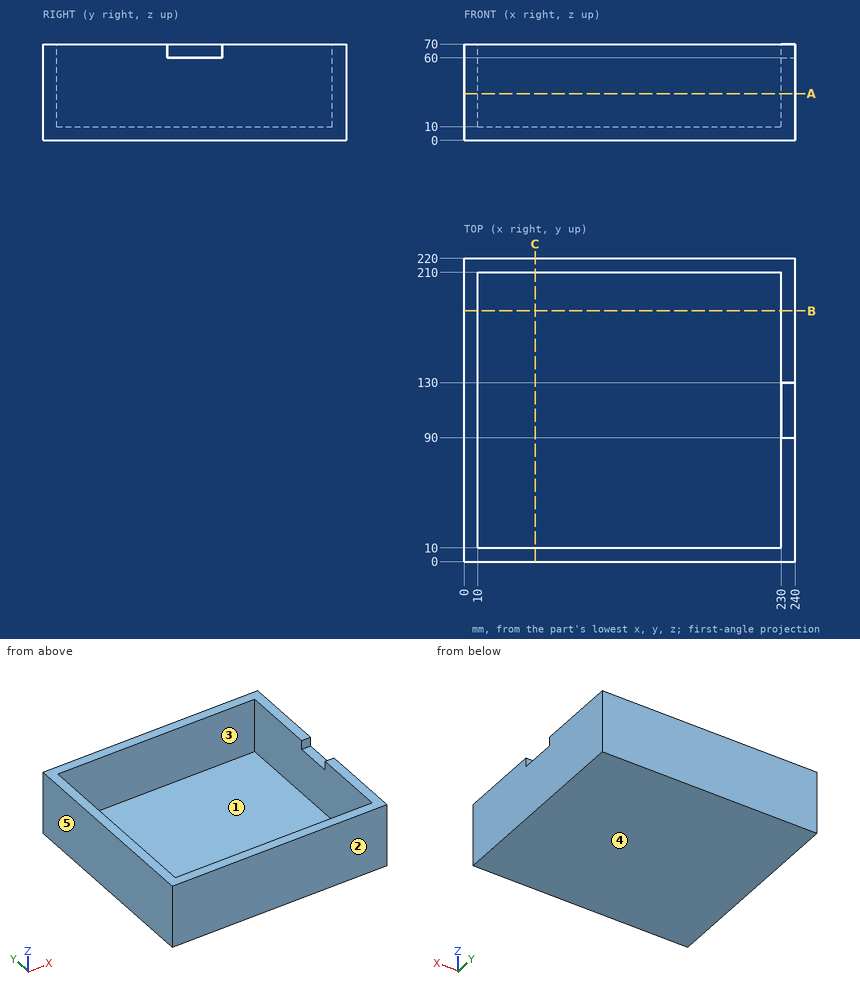
The figure shows three views and two pictorial views of one solid part (mm, origin at its lowest corner). Answer the questions. A direction names the side the tool comes from. Give positions to 0.01 mm unless a question says otherwise; leave off trailing zeros. Order: outer loops, then holes, each group sorted by start corner. A loop starts at its lowest first (then second) coordinate and runs counter-clockwise, first axis right, second up. Notation, with made-up numbers: (6, 50.25) -> (31, 50.25) arc R30 ccw to (31, 88.25) -> close; hole circle Ø10 at (20.5, -25). An arc over 180 degrees is marked (long way). Answer as a JSON object with one key per item and string values. Group by question number.
Item 1: The part is cut by section B-B on y = 182. Write down the section's boundary in (x, z), and give its area (3 significant figures).
Item 2: The part is cut by section A-A on z = 34. Write down the section's boundary in (x, y).
Item 3: Determine the mould class of the marked faces 3, 4 and 5 for opening direction X: pulls with the +X half, pulls with the -X half, needs draft (parallel to the pull), parting line crosses it, or undercut.
Item 4: Consider L1, parallel to X at y = 117, z = 39; L2, parallel to Y at x = 208.5, z = 25; L3, parallel to Z at x = 178, y = 65.5. Determine where each line is inside the solid, lowest interval first. Write a range as from..to.
Item 5: A tool of negligible diameter and unlimited length cuts with its end or side. For the marked faces 1 and 2, from which of +Z, -Z, +X, -X, +Y, -Y can it reach the whole face along a straight path? Write none if from no direction.
Item 6: Flat-ended cylindrical pins translate along their axes: pin 1 (2 mm diameter, centred on x = 25, y = 195, fed in from +Z); pin 2 (3 mm diameter, centred on x = 237, y = 107.5, fed in from +Z). Find the tip coordinate at first contact, or state that the pin passes through.
Item 7: The part is cut by section C-C on x = 51.5. Write down the section's boundary in (y, z).
Result set:
{
 "1": {"outline": "(0, 0) -> (240, 0) -> (240, 70) -> (230, 70) -> (230, 10) -> (10, 10) -> (10, 70) -> (0, 70) -> close", "area": "3,600 mm²"},
 "2": {"outline": "(0, 0) -> (240, 0) -> (240, 220) -> (0, 220) -> close; hole (10, 10) -> (230, 10) -> (230, 210) -> (10, 210) -> close"},
 "3": {"face 3": "undercut", "face 4": "needs draft", "face 5": "pulls with the -X half"},
 "4": {"L1": "0..10, 230..240", "L2": "0..10, 210..220", "L3": "0..10"},
 "5": {"face 1": "+Z", "face 2": "+Z, -Z, +X, -X, -Y"},
 "6": {"pin 1": "z = 10", "pin 2": "z = 60"},
 "7": {"outline": "(0, 0) -> (220, 0) -> (220, 70) -> (210, 70) -> (210, 10) -> (10, 10) -> (10, 70) -> (0, 70) -> close"}
}
